Could you check a few things on this model? Use its own coordinates, in mm. Face numbers are marked on the shaded views. A direction names the side the tool comes from. Give positions to 0.01 mm unless a question says otherwise; leave off trailing zeros. Order: outer loops, then holes, each group sorted by start corner. A loop starts at its lowest first (then second) coordinate and runs counter-clockwise, first axis right, second up. Notation, with made-up numbers: (56.5, -10) - (69.5, -10) arc R16 ccw to (69.5, 20) - close; hole circle Ø7 at (-5.75, -26). An arc over 180 degrees is marked (long way). One line per question, with ' | ' between items. Start each with the question number.
1. For P1, Ø2, axis at x = 2.5, z = 1.5, coming from the +Y side; P2, Ø3.5, axis at x = 18.5, z = -0.5, coming from the +Y side, each with a flat end and sliding along its axis, tell me the tip position at first contact or that it passes through.
2. If we mould it in two halves opening along X, with no side actions, what happens to the marked faces 4, 5, 6 and 7? For each: released by +X, released by -X, zero draft, split by the parting line, or undercut.
3. Which directions (+Z, -Z, +X, -X, +Y, -Y) give clear straight access to the entire face, cutting with the end or side of a thin tool? Please do the marked faces 1, 2 and 3.
4. I need wall thicknesses on probe 1 along Y at (x, z) = (-11, 2.5); probe 2 along Y at (x, z) = (-17.5, -0.5); probe 3 along X at (y, z) = (-14.5, -0.25). Which ranges of each line are inside material? Lowest first, please. Write a range as from..to.
5. Imagine slicing it at B-B (y = 24.5). Please give me the cut outline in (x, z).
6. Imagine slicing it at A-A (x = -7). Please give me the cut outline in (y, z).
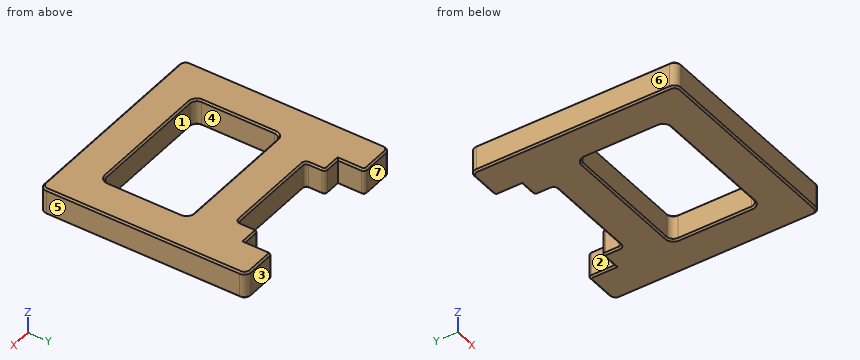
Autodesk Inventor part; units mm, degrees
ref_plane "YZ Plane" through (0, 0, 0) normal (1, 0, 0) x (0, 1, 0)
ref_plane "XZ Plane" through (0, 0, 0) normal (0, 1, 0) x (-1, 0, 0)
ref_plane "XY Plane" through (0, 0, 0) normal (0, 0, 1) x (1, 0, 0)
sketch "スケッチ1" plane through (0, 0, 0) normal (0, 0, 1) x (1, 0, 0)
  line L0 (-31, -31) -> (31, -31)
  line L1 (31, -31) -> (31, 31)
  line L2 (31, 31) -> (-31, 31)
  line L3 (-31, 31) -> (-31, -31)
  line L4 (-31, -31) -> (31, 31) construction
  line L5 (31, -31) -> (-31, 31) construction
  point P0 (0, 0)
  dimension "d0" = 62
  dimension "d1" = 62
extrude "押し出し1" add sketch "スケッチ1" along normal mid plane 8
sketch "スケッチ2" plane through (0, 0, 4) normal (0, 0, 1) x (1, 0, 0)
  line L0 (-20, 23) -> (20, 23)
  line L1 (20, 23) -> (20, 31)
  line L2 (20, 31) -> (-20, 31)
  line L3 (-20, 31) -> (-20, 23)
  line L4 (-20, 23) -> (20, 31) construction
  line L5 (20, 23) -> (-20, 31) construction
  line L6 (31, 31) -> (-31, 31)
  line L7 (-14.5, 17) -> (14.5, 17)
  line L8 (14.5, 17) -> (14.5, 23)
  line L9 (14.5, 23) -> (-14.5, 23)
  line L10 (-14.5, 23) -> (-14.5, 17)
  line L11 (-14.5, 17) -> (14.5, 23) construction
  line L12 (14.5, 17) -> (-14.5, 23) construction
  point P0 (0, 0)
  point P1 (0, 27)
  point P2 (0, 27)
  point P3 (0, 20)
  point P4 (0, 20)
  point P5 (0, 27)
  point P6 (14.5, 23)
  dimension "d4" = 40
  dimension "d5" = 8
  dimension "d14" = 29
  dimension "d15" = 6
extrude "押し出し2" cut sketch "スケッチ2" against normal blind 10
sketch "スケッチ3" plane through (0, 0, 4) normal (0, 0, 1) x (1, 0, 0)
  line L0 (-20, -20) -> (20, -20)
  line L1 (20, -20) -> (20, 6)
  line L2 (20, 6) -> (-20, 6)
  line L3 (-20, 6) -> (-20, -20)
  line L4 (-20, -20) -> (20, 6) construction
  line L5 (20, -20) -> (-20, 6) construction
  line L6 (-31, 31) -> (-31, -31)
  line L7 (-31, -31) -> (31, -31)
  line L8 (14.5, 17) -> (-14.5, 17)
  point P0 (0, 0)
  point P1 (0, -7)
  point P2 (0, -7)
  dimension "d10" = 11
  dimension "d11" = 11
  dimension "d16" = 11
extrude "押し出し3" cut sketch "スケッチ3" against normal through all
fillet "フィレット2" radius 1 6 edges at (-14.5, 23, 0) (-14.5, 17, 0) (14.5, 17, 0) (14.5, 23, 0) (-20, 31, 0) (20, 31, 0)
fillet "フィレット3" radius 2 4 edges at (-31, 31, 0) (-31, -31, 0) (31, -31, 0) (31, 31, 0)
fillet "フィレット4" radius 2 4 edges at (-20, 6, 0) (-20, -20, 0) (20, -20, 0) (20, 6, 0)
chamfer "面取り1" distance 0.5 angle 45 60 edges at (31, 0, -4) (30.4142, -30.4142, -4) (0, -31, -4) (-30.4142, -30.4142, -4) (-31, 0, -4) (-30.4142, 30.4142, -4) (-25, 31, -4) (-20.2929, 30.7071, -4) (-20, 26.5, -4) (30.4142, 30.4142, -4) (25, 31, -4) (20.2929, 30.7071, -4) (20, 26.5, -4) (31, 0, 4) (30.4142, 30.4142, 4) (25, 31, 4) (20.2929, 30.7071, 4) (20, 26.5, 4) (30.4142, -30.4142, 4) (0, -31, 4) (-30.4142, -30.4142, 4) (-31, 0, 4) (-30.4142, 30.4142, 4) (-25, 31, 4) (-20.2929, 30.7071, 4) (-20, 26.5, 4) (17.75, 23, -4) (14.7929, 22.7071, -4) (14.5, 20, -4) (14.2071, 17.2929, -4) (0, 17, -4) (-14.2071, 17.2929, -4) (-14.5, 20, -4) (-14.7929, 22.7071, -4) (-17.75, 23, -4) (17.75, 23, 4) (14.7929, 22.7071, 4) (14.5, 20, 4) (14.2071, 17.2929, 4) (0, 17, 4) (-14.2071, 17.2929, 4) (-14.5, 20, 4) (-14.7929, 22.7071, 4) (-17.75, 23, 4) (0, 6, 4) (19.4142, 5.4142, 4) (20, -7, 4) (19.4142, -19.4142, 4) (0, -20, 4) (-19.4142, -19.4142, 4) (-20, -7, 4) (-19.4142, 5.4142, 4) (0, -20, -4) (19.4142, -19.4142, -4) (20, -7, -4) (19.4142, 5.4142, -4) (0, 6, -4) (-19.4142, 5.4142, -4) (-20, -7, -4) (-19.4142, -19.4142, -4)
properties part number "scara-base29" material "ABS プラスチック"
Results found:
1) P1: stops at y = 17 | P2: stops at y = 30.66
2) face 4: undercut | face 5: released by +X | face 6: released by -X | face 7: zero draft
3) face 1: +Z, -Z | face 2: +Z, -Z, +Y | face 3: +Z, -Z, +X, -X, +Y
4) probe 1: y = -31..-20, 6..17 | probe 2: y = -31..-20, 6..23 | probe 3: x = -31..-20, 20..31
5) outline: (-31, -3.5) - (-30.5, -4) - (-20.5, -4) - (-20, -3.5) - (-20, 3.5) - (-20.5, 4) - (-30.5, 4) - (-31, 3.5) - close; (20, -3.5) - (20.5, -4) - (30.5, -4) - (31, -3.5) - (31, 3.5) - (30.5, 4) - (20.5, 4) - (20, 3.5) - close
6) outline: (-31, -3.5) - (-30.5, -4) - (-20.5, -4) - (-20, -3.5) - (-20, 3.5) - (-20.5, 4) - (-30.5, 4) - (-31, 3.5) - close; (6, -3.5) - (6.5, -4) - (16.5, -4) - (17, -3.5) - (17, 3.5) - (16.5, 4) - (6.5, 4) - (6, 3.5) - close
